Could you check a few things on this model? Use its own coordinates, in mm. A direction names the side the tool comes from. Give positions to 0.01 mm unless a question says otherwise; leave off trailing zeros. Order: outer loops, then holes, each group sorted by start corner. A loop starts at its lowest first (then second) coordinate and runs counter-clockwise, first axis right, second up. Notation, with made-up numbers: (-24.75, -29) - (20.25, -29) arc R17 cw to (20.25, -2) - close; hole circle Ø6 at (55, 63.5). An arc over 180 degrees is marked (long way). Put each result on its own line as item: value.
from build123d import *

# Parameters (mm, degrees)
BOSS_EXTRUDE3_DEPTH = 20
SKETCH3_R           = 1.25
CUT_EXTRUDE1_DEPTH  = 66.239941753
SKETCH5_R           = 1.25
CUT_EXTRUDE2_DEPTH  = 56.283360969


with BuildPart() as part:
    # Sketch2 → Boss-Extrude3 (new body)
    with BuildSketch(Plane.XY):
        with BuildLine():
            Line((-20, 0), (20, 0))
            Line((20, 0), (20, 45))
            ThreePointArc((20, 45), (17.5, 47.5), (15, 45))
            Line((15, 45), (15, 5))
            Line((15, 5), (-15, 5))
            Line((-15, 5), (-15, 45))
            ThreePointArc((-15, 45), (-17.5, 47.5), (-20, 45))
            Line((-20, 45), (-20, 0))
        make_face()
    extrude(amount=BOSS_EXTRUDE3_DEPTH)

    # Sketch3 → Cut-Extrude1 (cut, through all)
    with BuildSketch(Plane.ZY.offset(20)):
        with Locations(Location((10, 38.137651085, 0), (0, 0, 270))):
            Circle(SKETCH3_R)
    extrude(amount=-CUT_EXTRUDE1_DEPTH, mode=Mode.SUBTRACT)

    # Sketch5 → Cut-Extrude2 (cut, through all)
    with BuildSketch(Plane.XZ):
        with Locations((0, 10.783115236)):
            Circle(SKETCH5_R)
    extrude(amount=-CUT_EXTRUDE2_DEPTH, mode=Mode.SUBTRACT)


solid = part.part
1) Suppose I cut it at B-B, the plane y = 44. List the corners of the cut face in (x, z) for me.
Filled in:
outline: (-20, 0) - (-15, 0) - (-15, 20) - (-20, 20) - close; (15, 0) - (20, 0) - (20, 20) - (15, 20) - close
2) Suppose I cut it at D-D, the plane x = 6.5. List the corners of the cut face in (y, z) for me, and give its area (3 significant figures).
Filled in:
outline: (0, 0) - (5, 0) - (5, 20) - (0, 20) - close
area: 100 mm^2
3) Which directions (+Z, -Z, +X, -X, +Y, -Y) give clear straight access to the entire face, cutting with the end or side of a thin tool? Please do faces 1 (the flat face through (15, 25, 10)), 2 (the cylindrical face through (-0.271, 2.465, 9.563)).
Filled in:
face 1: +Z, -Z, +Y
face 2: +Y, -Y
4) If I drill on line 1 (X direction, y = 27.5, z = 17); line 2 (Z direction, x = 0, y = 3.2); line 3 (Y direction, x = 1.5, z = 2.25), over which ranges is the centre line in solid material (lowest first)? Write a range as [from, to].
Filled in:
line 1: x = [-20, -15], [15, 20]
line 2: z = [0, 9.53], [12.03, 20]
line 3: y = [0, 5]
5) We'd pull the mould along X, two halves only. Please class faces 3 (the flat face through (-0.1, 4.5, 20)), 4 (the flat face through (20, 22, 10)), 5 (the cylindrical face through (-17.4, 47.5, 9.9)): pulls with the +X half, pulls with the -X half, needs draft (parallel to the pull), parting line crosses it, or undercut.
Filled in:
face 3: needs draft
face 4: pulls with the +X half
face 5: undercut
6) I'm going to push flat-ended pins straight in: pin 1 (2 mm diameter, centred on x = -9, z = 14.5, fed in from +Y); pin 2 (2 mm diameter, centred on y = 38.14, z = 10, fed in from +X). Where does each tip first touch, or does it pass through?
Filled in:
pin 1: stops at y = 5
pin 2: passes through
7) Suppose I cut it at A-A, the plane x = 0. List the corners of the cut face in (y, z) for me, and give its area (3 significant figures).
Filled in:
outline: (0, 0) - (5, 0) - (5, 9.53) - (0, 9.53) - close; (0, 12.03) - (5, 12.03) - (5, 20) - (0, 20) - close
area: 87.5 mm^2
8) Suppose I cut it at C-C, the plane z = 6.75. List the corners of the cut face in (x, y) for me.
Filled in:
outline: (-20, 0) - (20, 0) - (20, 45) arc R2.5 ccw to (15, 45) - (15, 5) - (-15, 5) - (-15, 45) arc R2.5 ccw to (-20, 45) - close
